Check sheet for the drawn part. Datum: minimum x, y, z corner. Units: mm. A direction names the side the tool comes from. Coordinates: 2 decimals unless noted, no trailing zeros. Loops run counter-clockwise (first coordinate to the right, second up) from the corner with the lowest first, then second, coordinate; pieces in that order, holes last.
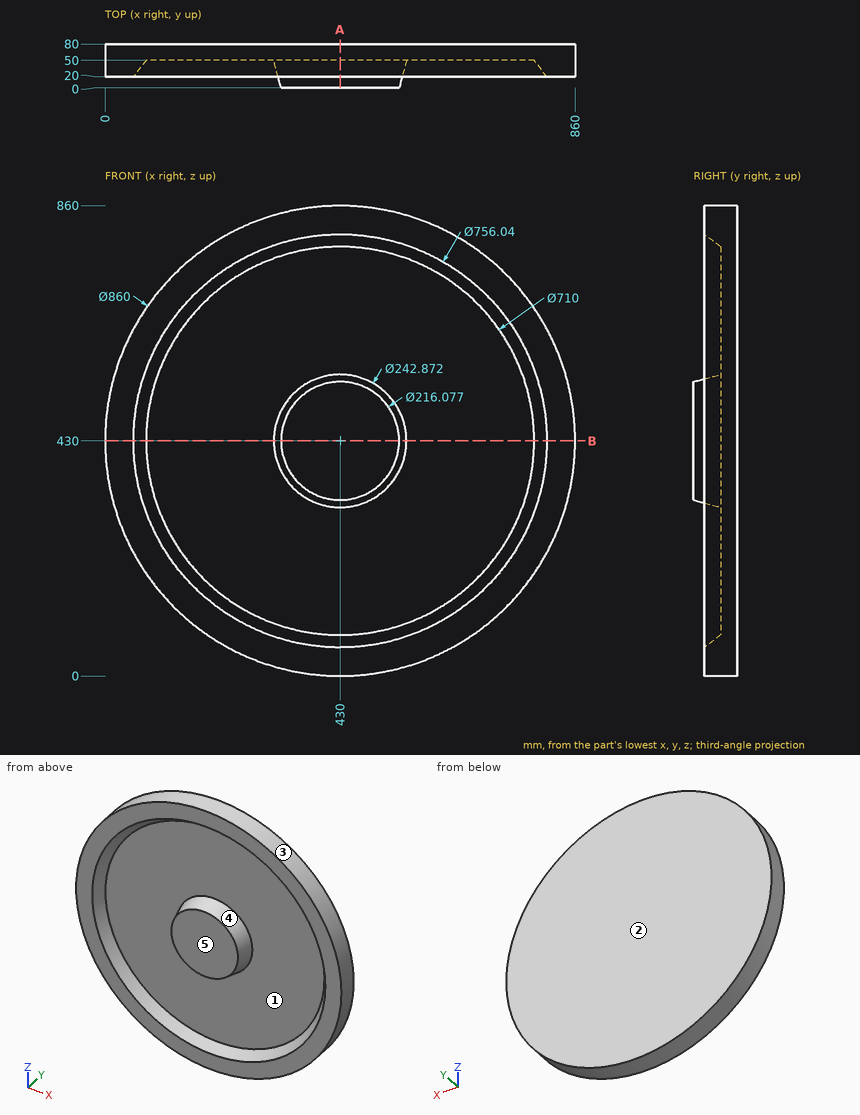
1) Depth check by flat-ended pin: pin 1 (1 mm diameter, centred on y = 55.5, z = 113, fed in from +X); pin 2 (4 mm diameter, centred on x = 421, y = 14.5, fed in from +Z); pin 3 (5 mm diameter, centred on x = 565, z = 347.5, fed in from -Y). Enter the tip coordinate at first touch or a pass-through.
Answer sheet:
pin 1: stops at x = 721.08
pin 2: stops at z = 542.12
pin 3: stops at y = 50
2) Mould release check, pull along X, two halves, no side actions. Record for the marked faces 3, 4 and 5: +X half, -X half, draft (parallel to the pull), parting line (faces both ways), or undercut.
Answer sheet:
face 3: parting line
face 4: undercut
face 5: draft
3) Section check B-B on z = 430. Enter the section's corners in (x, y).
Answer sheet:
outline: (0, 20) - (51.98, 20) - (75, 50) - (308.56, 50) - (321.96, 0) - (538.04, 0) - (551.44, 50) - (785, 50) - (808.02, 20) - (860, 20) - (860, 80) - (0, 80) - close
4) Scan lines: line 1 (X direction, y = 27.5, z = 457.5); line 2 (X direction, y = 36, z = 493.5) (1 decimal); line 3 (Z direction, x = 376, y = 37) (1 decimal). Record each from-to range of solid material in increasing order.
Answer sheet:
line 1: x = 0.88 to 58.75, 317.92 to 542.08, 801.25 to 859.12
line 2: x = 4.7 to 69.8, 330.9 to 529.1, 790.2 to 855.3
line 3: z = 3.4 to 69, 325.1 to 534.9, 791 to 856.6
5) Section check A-A on x = 430. Enter the section's corners in (y, z), plus the area to 3 significant figures.
Answer sheet:
outline: (0, 321.96) - (50, 308.56) - (50, 75) - (20, 51.98) - (20, 0) - (80, 0) - (80, 860) - (20, 860) - (20, 808.02) - (50, 785) - (50, 551.44) - (0, 538.04) - close
area: 41,100 mm2
6) Set-up check for the marked faces 1 and 2: record each of +Z, -Z, +X, -X, +Y, -Y from which the full face is reachable in a straight line by a thin tool's end or side.
Answer sheet:
face 1: -Y
face 2: +Z, -Z, +X, -X, +Y
